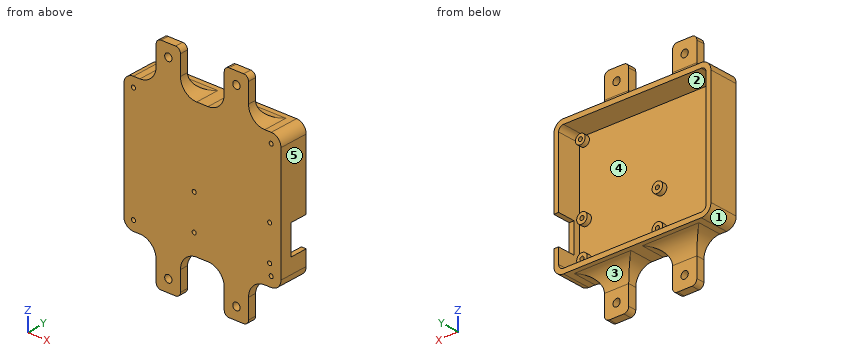
from build123d import *

# Parameters (mm, degrees)
BOSS_EXTRUDE1_DEPTH = 3
BOSS_EXTRUDE2_START = 15
BOSS_EXTRUDE2_DEPTH = 15
BOSS_EXTRUDE3_START = 3
SKETCH1_5_R         = 1.25
SKETCH1_5_R_2       = 3.25
BOSS_EXTRUDE3_DEPTH = 3
SKETCH1_6_R         = 1.25
CUT_EXTRUDE1_DEPTH  = 124.701253025
CUT_EXTRUDE2_REACH  = 127.996
SKETCH3_W           = 18.2
SKETCH3_H           = 11
SKETCH4_R           = 2.25
BOSS_EXTRUDE4_DEPTH = 5
FILLET1_R           = 10


with BuildPart() as part:
    # Sketch1 → Boss-Extrude1 (new body)
    with BuildSketch(Plane(origin=(0, 0, 0), x_dir=(1, 0, 0), z_dir=(0, 1, 0))):
        with BuildLine():
            Line((-3, 3), (-88, 3))
            ThreePointArc((-88, 3), (-92.242640687, 1.242640687), (-94, -3))
            Line((-94, -3), (-94, -73))
            ThreePointArc((-94, -73), (-92.242640687, -77.242640687), (-88, -79))
            Line((-88, -79), (-3, -79))
            ThreePointArc((-3, -79), (1.242640687, -77.242640687), (3, -73))
            Line((3, -73), (3, -3))
            ThreePointArc((3, -3), (1.242640687, 1.242640687), (-3, 3))
        make_face()
    extrude(amount=-BOSS_EXTRUDE1_DEPTH)

    # Sketch1_4 → Boss-Extrude2 (add)
    with BuildSketch(Plane(origin=(0, 0, 0), x_dir=(1, 0, 0), z_dir=(0, 1, 0)).offset(BOSS_EXTRUDE2_START)):
        with BuildLine():
            ThreePointArc((-3, 3), (1.242640687, 1.242640687), (3, -3))
            Line((3, -3), (3, -73))
            ThreePointArc((3, -73), (1.242640687, -77.242640687), (-3, -79))
            Line((-3, -79), (-88, -79))
            ThreePointArc((-88, -79), (-92.242640687, -77.242640687), (-94, -73))
            Line((-94, -73), (-94, -3))
            ThreePointArc((-94, -3), (-92.242640687, 1.242640687), (-88, 3))
            Line((-88, 3), (-3, 3))
        make_face()
        with BuildLine():
            Line((-3, 0), (-88, 0))
            ThreePointArc((-88, 0), (-90.121320344, -0.878679656), (-91, -3))
            Line((-91, -3), (-91, -73))
            ThreePointArc((-91, -73), (-90.121320344, -75.121320344), (-88, -76))
            Line((-88, -76), (-3, -76))
            ThreePointArc((-3, -76), (-0.878679656, -75.121320344), (0, -73))
            Line((0, -73), (0, -3))
            ThreePointArc((0, -3), (-0.878679656, -0.878679656), (-3, 0))
        make_face(mode=Mode.SUBTRACT)
    extrude(amount=-BOSS_EXTRUDE2_DEPTH)

    # Sketch1_5 → Boss-Extrude3 (add)
    # profile 1 of 8: a face of its own
    with BuildSketch(Plane(origin=(0, 0, 0), x_dir=(1, 0, 0), z_dir=(0, 1, 0)).offset(BOSS_EXTRUDE3_START)):
        with BuildLine():
            ThreePointArc((-85, -3), (-85.878679656, -0.878679656), (-88, 0))
            ThreePointArc((-88, 0), (-90.121320344, -0.878679656), (-91, -3))
            ThreePointArc((-91, -3), (-88, -6), (-85, -3))
        make_face()
        with Locations(Location((-88, -3, 0), (0, 0, 270))):
            Circle(SKETCH1_5_R, mode=Mode.SUBTRACT)
    # profile 2 of 8: a face of its own
    with BuildSketch(Plane(origin=(0, 0, 0), x_dir=(1, 0, 0), z_dir=(0, 1, 0)).offset(BOSS_EXTRUDE3_START)):
        with Locations(Location((-50.53, -9.5, 0), (0, 0, 90))):
            Circle(SKETCH1_5_R_2)
        with Locations(Location((-50.53, -9.5, 0), (0, 0, 270))):
            Circle(SKETCH1_5_R, mode=Mode.SUBTRACT)
    # profile 3 of 8: a face of its own
    with BuildSketch(Plane(origin=(0, 0, 0), x_dir=(1, 0, 0), z_dir=(0, 1, 0)).offset(BOSS_EXTRUDE3_START)):
        with Locations(Location((-50.53, -31, 0), (0, 0, 90))):
            Circle(SKETCH1_5_R_2)
        with Locations(Location((-50.53, -31, 0), (0, 0, 270))):
            Circle(SKETCH1_5_R, mode=Mode.SUBTRACT)
    # profile 4 of 8: a face of its own
    with BuildSketch(Plane(origin=(0, 0, 0), x_dir=(1, 0, 0), z_dir=(0, 1, 0)).offset(BOSS_EXTRUDE3_START)):
        with BuildLine():
            ThreePointArc((0, -3), (-0.878679656, -0.878679656), (-3, 0))
            ThreePointArc((-3, 0), (-5.121320344, -5.121320344), (0, -3))
        make_face()
        with Locations(Location((-3, -3, 0), (0, 0, 270))):
            Circle(SKETCH1_5_R, mode=Mode.SUBTRACT)
    # profile 5 of 8: a face of its own
    with BuildSketch(Plane(origin=(0, 0, 0), x_dir=(1, 0, 0), z_dir=(0, 1, 0)).offset(BOSS_EXTRUDE3_START)):
        with Locations(Location((-3.99, -9.5, 0), (0, 0, 90))):
            Circle(SKETCH1_5_R_2)
        with Locations(Location((-3.99, -9.5, 0), (0, 0, 270))):
            Circle(SKETCH1_5_R, mode=Mode.SUBTRACT)
    # profile 6 of 8: a face of its own
    with BuildSketch(Plane(origin=(0, 0, 0), x_dir=(1, 0, 0), z_dir=(0, 1, 0)).offset(BOSS_EXTRUDE3_START)):
        with Locations(Location((-3.99, -31, 0), (0, 0, 90))):
            Circle(SKETCH1_5_R_2)
        with Locations(Location((-3.99, -31, 0), (0, 0, 270))):
            Circle(SKETCH1_5_R, mode=Mode.SUBTRACT)
    # profile 7 of 8: a face of its own
    with BuildSketch(Plane(origin=(0, 0, 0), x_dir=(1, 0, 0), z_dir=(0, 1, 0)).offset(BOSS_EXTRUDE3_START)):
        with BuildLine():
            ThreePointArc((-3, -76), (-0.878679656, -75.121320344), (0, -73))
            ThreePointArc((0, -73), (-5.121320344, -70.878679656), (-3, -76))
        make_face()
        with Locations(Location((-3, -73, 0), (0, 0, 270))):
            Circle(SKETCH1_5_R, mode=Mode.SUBTRACT)
    # profile 8 of 8: a face of its own
    with BuildSketch(Plane(origin=(0, 0, 0), x_dir=(1, 0, 0), z_dir=(0, 1, 0)).offset(BOSS_EXTRUDE3_START)):
        with BuildLine():
            ThreePointArc((-85, -73), (-88, -70), (-91, -73))
            ThreePointArc((-91, -73), (-90.121320344, -75.121320344), (-88, -76))
            ThreePointArc((-88, -76), (-85.878679656, -75.121320344), (-85, -73))
        make_face()
        with Locations(Location((-88, -73, 0), (0, 0, 270))):
            Circle(SKETCH1_5_R, mode=Mode.SUBTRACT)
    extrude(amount=-BOSS_EXTRUDE3_DEPTH)

    # Sketch1_6 → Cut-Extrude1 (cut, through all)
    with BuildSketch(Plane(origin=(0, 0, 0), x_dir=(1, 0, 0), z_dir=(0, 1, 0))):
        with Locations(Location((-3.99, -9.5, 0), (0, 0, 270))):
            Circle(SKETCH1_6_R)
        with Locations(Location((-50.53, -9.5, 0), (0, 0, 270))):
            Circle(SKETCH1_6_R)
        with Locations(Location((-3.99, -31, 0), (0, 0, 270))):
            Circle(SKETCH1_6_R)
        with Locations(Location((-50.53, -31, 0), (0, 0, 270))):
            Circle(SKETCH1_6_R)
        with Locations(Location((-3, -3, 0), (0, 0, 270))):
            Circle(SKETCH1_6_R)
        with Locations(Location((-88, -3, 0), (0, 0, 270))):
            Circle(SKETCH1_6_R)
        with Locations(Location((-88, -73, 0), (0, 0, 270))):
            Circle(SKETCH1_6_R)
        with Locations(Location((-3, -73, 0), (0, 0, 270))):
            Circle(SKETCH1_6_R)
    extrude(amount=-CUT_EXTRUDE1_DEPTH, mode=Mode.SUBTRACT)

    # Sketch3 → Cut-Extrude2 (cut, up to next)
    with BuildSketch(Plane(origin=(3, 0, 0), x_dir=(0, 0, -1), z_dir=(1, 0, 0)), mode=Mode.PRIVATE) as cut_extrude2_sk1:
        with Locations((-21.42, 9.5)):
            Rectangle(SKETCH3_W, SKETCH3_H)
    cut_extrude2_tool1 = extrude(cut_extrude2_sk1.sketch, amount=-CUT_EXTRUDE2_REACH, mode=Mode.PRIVATE) & part.part
    add(cut_extrude2_tool1.solids().sort_by_distance((3, 9.5, 21.42))[0], mode=Mode.SUBTRACT)

    # Sketch4 → Boss-Extrude4 (add)
    # profile 1 of 4: a face of its own
    with BuildSketch(Plane.XZ.offset(3)):
        with BuildLine():
            Line((-17, 79), (-32, 79))
            Line((-32, 79), (-32, 101))
            ThreePointArc((-32, 101), (-31.121320344, 103.121320344), (-29, 104))
            Line((-29, 104), (-20, 104))
            ThreePointArc((-20, 104), (-17.878679656, 103.121320344), (-17, 101))
            Line((-17, 101), (-17, 79))
        make_face()
        with Locations(Location((-24.5, 96.5, 0), (0, 0, 270))):
            Circle(SKETCH4_R, mode=Mode.SUBTRACT)
    # profile 2 of 4: a face of its own
    with BuildSketch(Plane.XZ.offset(3)):
        with BuildLine():
            Line((-17, -3), (-32, -3))
            Line((-32, -3), (-32, -25))
            ThreePointArc((-32, -25), (-31.121320344, -27.121320344), (-29, -28))
            Line((-29, -28), (-20, -28))
            ThreePointArc((-20, -28), (-17.878679656, -27.121320344), (-17, -25))
            Line((-17, -25), (-17, -3))
        make_face()
        with Locations(Location((-24.5, -20.5, 0), (0, 0, 270))):
            Circle(SKETCH4_R, mode=Mode.SUBTRACT)
    # profile 3 of 4: a face of its own
    with BuildSketch(Plane.XZ.offset(3)):
        with BuildLine():
            Line((-59, 79), (-74, 79))
            Line((-74, 79), (-74, 101))
            ThreePointArc((-74, 101), (-73.121320344, 103.121320344), (-71, 104))
            Line((-71, 104), (-62, 104))
            ThreePointArc((-62, 104), (-59.878679656, 103.121320344), (-59, 101))
            Line((-59, 101), (-59, 79))
        make_face()
        with Locations(Location((-66.5, 96.5, 0), (0, 0, 270))):
            Circle(SKETCH4_R, mode=Mode.SUBTRACT)
    # profile 4 of 4: a face of its own
    with BuildSketch(Plane.XZ.offset(3)):
        with BuildLine():
            Line((-59, -3), (-74, -3))
            Line((-74, -3), (-74, -25))
            ThreePointArc((-74, -25), (-73.121320344, -27.121320344), (-71, -28))
            Line((-71, -28), (-62, -28))
            ThreePointArc((-62, -28), (-59.878679656, -27.121320344), (-59, -25))
            Line((-59, -25), (-59, -3))
        make_face()
        with Locations(Location((-66.5, -20.5, 0), (0, 0, 270))):
            Circle(SKETCH4_R, mode=Mode.SUBTRACT)
    extrude(amount=-BOSS_EXTRUDE4_DEPTH)

    # Fillet1
    fillet1_edges = [part.edges().sort_by_distance(p)[0] for p in [
        (-24.5, 2, 79),
        (-17, -0.5, 79),
        (-32, -0.5, 79),
        (-17, -0.5, -3),
        (-24.5, 2, -3),
        (-32, -0.5, -3),
        (-66.5, 2, 79),
        (-59, -0.5, 79),
        (-74, -0.5, 79),
        (-59, -0.5, -3),
        (-66.5, 2, -3),
        (-74, -0.5, -3),
    ]]
    fillet(fillet1_edges, radius=FILLET1_R)


solid = part.part
Could you check a few things on this model? Use its own coordinates, in mm. Face numbers are marked on the shaded views. A direction names the side the tool comes from. Give positions to 0.01 mm unless a question says otherwise; leave off trailing zeros. Loops run counter-clockwise (first coordinate to the right, second up) from the corner with the lowest first, then second, coordinate; pieces in that order, holes last. Notation, with made-up numbers: (43, 10.25) -> (47, 10.25) arc R11 ccw to (47, 27.25) -> close; hole circle Ø4 at (59, 60). An arc over 180 degrees is marked (long way). Return JSON: item names as keys, results as strings.
Item 1: If we section it at A-A on z = -20.5: List the corners of the cut face in (x, y) for me.
Geometry results:
{"outline": "(-74, -3) -> (-68.75, -3) -> (-68.75, 2) -> (-74, 2) -> close; (-64.25, -3) -> (-59, -3) -> (-59, 2) -> (-64.25, 2) -> close; (-32, -3) -> (-26.75, -3) -> (-26.75, 2) -> (-32, 2) -> close; (-22.25, -3) -> (-17, -3) -> (-17, 2) -> (-22.25, 2) -> close"}
Item 2: I'm going to push flat-ended pins straight in: pin 1 (4 mm diameter, centred on x = -68, z = 24.5, fed in from +Y); pin 2 (3 mm diameter, centred on x = -82.5, y = 4, fed in from +Z); pin 3 (1.5 mm diameter, centred on x = -3.99, z = 9.5, fed in from +Y); pin 4 (1.8 mm diameter, centred on x = -3, z = 3.5, fed in from +Y). Where does each tip first touch, or does it pass through?
Geometry results:
{"pin 1": "stops at y = 0", "pin 2": "stops at z = 79.46", "pin 3": "passes through", "pin 4": "stops at y = 3"}
Item 3: I need wall thicknesses on L1, parallel to X at y = 1.75, z = 31; L2, parallel to X at y = -1, z = 31; L3, parallel to X at y = -1.95, z = 96.5. Which ranges of each line are inside material? Lowest first, please. Write a range as from..to.
Geometry results:
{"L1": "x = -94..-91, -53.78..-51.78, -49.28..-47.28, -7.24..-5.24, -2.74..-0.74, 0..3", "L2": "x = -94..-51.78, -49.28..-5.24, -2.74..3", "L3": "x = -74..-68.75, -64.25..-59, -32..-26.75, -22.25..-17"}
Item 4: If we section it at B-B on z = 46.5: List the corners of the cut face in (x, y) for me, plus the area to 3 significant figures.
Geometry results:
{"outline": "(-94, -3) -> (3, -3) -> (3, 15) -> (0, 15) -> (0, 0) -> (-91, 0) -> (-91, 15) -> (-94, 15) -> close", "area": "381 mm²"}
Item 5: If we section it at C-C on z = 23.5: List the corners of the cut face in (x, y) for me, plus the area to 3 significant figures.
Geometry results:
{"outline": "(-94, -3) -> (3, -3) -> (3, 4) -> (0, 4) -> (0, 0) -> (-91, 0) -> (-91, 15) -> (-94, 15) -> close", "area": "348 mm²"}
Item 6: Which directions (+Z, -Z, +X, -X, +Y, -Y) give clear straight access to the entire face, cutting with the end or side of a thin tool? Please do the marked faces 1 and 2.
Geometry results:
{"face 1": "-Z, -X, +Y, -Y", "face 2": "+Y"}
Item 7: We'd pull the mould along X, two halves only. Please class the marked faces 3, 4 and 5: +X half, -X half, draft (parallel to the pull), parting line (faces both ways), or undercut.
Geometry results:
{"face 3": "draft", "face 4": "undercut", "face 5": "+X half"}
